from build123d import *

# Parameters (mm, degrees)
SKETCH_1_W      = 80
SKETCH_1_H      = 80
SKETCH_1_R      = 22.5
EXTRUDE_1_DEPTH = 15
FILLET_1_R      = 5
SKETCH_2_R      = 7.5
EXTRUDE_2_DEPTH = 70
FILLET_2_R      = 3


with BuildPart() as part:
    # 草圖1 → 填料-伸長1 (new body)
    with BuildSketch(Plane(origin=(0, 0, 0), x_dir=(1, 0, 0), z_dir=(0, 1, 0))):
        with Locations((11.024390244, -21.451219512)):
            Rectangle(SKETCH_1_W, SKETCH_1_H)
        with Locations(Location((11.024390244, -21.451219512, 0), (0, 0, 270))):
            Circle(SKETCH_1_R, mode=Mode.SUBTRACT)
    extrude(amount=EXTRUDE_1_DEPTH)

    # 圓角1
    fillet_1_edges = [part.edges().sort_by_distance(p)[0] for p in [
        (-28.975609756, 7.5, -18.548780488),
        (51.024390244, 7.5, -18.548780488),
        (51.024390244, 7.5, 61.451219512),
        (-28.975609756, 7.5, 61.451219512),
    ]]
    fillet(fillet_1_edges, radius=FILLET_1_R)

    # 草圖2 → 填料-伸長2 (add)
    with BuildSketch(Plane(origin=(0, 15, 0), x_dir=(1, 0, 0), z_dir=(0, 1, 0))):
        with Locations(Location((-16.475609756, 6.048780488, 0), (0, 0, 270))):
            Circle(SKETCH_2_R)
        with Locations(Location((38.524390244, 6.048780488, 0), (0, 0, 270))):
            Circle(SKETCH_2_R)
        with Locations(Location((38.524390244, -48.951219512, 0), (0, 0, 270))):
            Circle(SKETCH_2_R)
        with Locations(Location((-16.475609756, -48.951219512, 0), (0, 0, 270))):
            Circle(SKETCH_2_R)
    extrude(amount=EXTRUDE_2_DEPTH)

    # 圓角2
    fillet_2_edges = [part.edges().sort_by_distance(p)[0] for p in [
        (-16.475609756, 15, -13.548780488),
        (38.524390244, 15, -13.548780488),
        (38.524390244, 15, 41.451219512),
        (-16.475609756, 15, 41.451219512),
    ]]
    fillet(fillet_2_edges, radius=FILLET_2_R)


solid = part.part
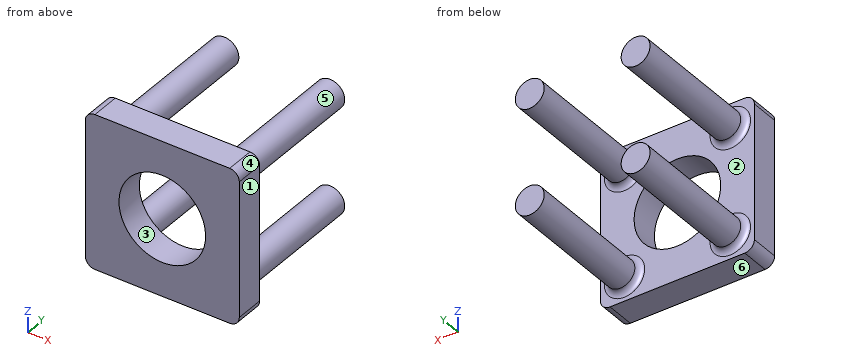
The listing builds one solid part. Answer for the finished solid, in the listing's coordinates (mm). Face numbers are marked on the shaded views. A direction names the side the tool comes from. Coordinates: 2 decimals unless noted, no trailing zeros. Write each loop counter-clockwise with the first axis right and the second up, starting at its lowest first coordinate (ties: lowest second). Pieces come first, ordered by that corner, then holes. Notation, with made-up numbers: (67.25, 31) -> (85.25, 31) arc R27 ccw to (85.25, 55) -> close; hole circle Ø1 at (59.5, -30). An arc over 180 degrees is marked (long way). One line per question, with ' | ' between items.
1. Section C-C (y = 80) is taken. Determine the outline of the cut face in (x, z).
Verdict:
outline: circle Ø15 at (-16.48, -6.05); circle Ø15 at (-16.48, 48.95); circle Ø15 at (38.52, -6.05); circle Ø15 at (38.52, 48.95)
2. Which of the six approach directions +Z, -Z, +X, -X, +Y, -Y give full straight-line access (tool end or side, diameter ignored) to the marked faces 1 and 2?
Verdict:
face 1: +Z, -Z, +X, +Y, -Y | face 2: +Y
3. For a pull along X with two mould halves and no side action, classify the marked faces 3, 4, 5 and 6 as released by +X, released by -X, zero draft, split by the parting line, or undercut.
Verdict:
face 3: undercut | face 4: released by +X | face 5: undercut | face 6: zero draft
4. Given pin 1 Ø1.5 at (y, z) = (62, -10) entering from -X; pin 2 Ø2 at (x, y) = (-12, 19.5) entering from -Z; pin 3 Ø8 at (x, y) = (-6.5, 30.5) entering from +Z; pin 4 Ø1.5 at (x, z) = (30.5, 27) entering from +Y, each flat-ended and moving along its own axis, determine where each tip first touches the part or whether it passes through.
Verdict:
pin 1: stops at x = -23.26 | pin 2: stops at z = -12.69 | pin 3: stops at z = 53.48 | pin 4: passes through
5. Section A-A (z = 37) is taken. Determine the outline of the cut face in (x, y).
Verdict:
outline: (-28.98, 0) -> (-5.24, 0) -> (-5.24, 15) -> (-28.98, 15) -> close; (27.29, 0) -> (51.02, 0) -> (51.02, 15) -> (27.29, 15) -> close
6. Straight lines are drawn through the part: line 1 (X direction, y = 8, z = 2.5); line 2 (Y direction, x = -6.5, z = 6); line 3 (X direction, y = 39.5, z = -12). For each, find the intervals that lie inside material, in ascending order.
Verdict:
line 1: x = -28.98 to -1.1, 23.15 to 51.02 | line 2: y = 0 to 15 | line 3: x = -21.04 to -11.91, 33.96 to 43.09
7. Section B-B (x = 23.5) is taken. Determine the outline of the cut face in (y, z), and give its area (3 significant figures).
Verdict:
outline: (0, -18.55) -> (15, -18.55) -> (15, 2.73) -> (0, 2.73) -> close; (0, 40.18) -> (15, 40.18) -> (15, 61.45) -> (0, 61.45) -> close | area: 638 mm^2
8. Section D-D (y = 10) is taken. Determine the outline of the cut face in (x, z), and give its area (3 significant figures).
Verdict:
outline: (-28.98, -13.55) arc R5 ccw to (-23.98, -18.55) -> (46.02, -18.55) arc R5 ccw to (51.02, -13.55) -> (51.02, 56.45) arc R5 ccw to (46.02, 61.45) -> (-23.98, 61.45) arc R5 ccw to (-28.98, 56.45) -> close; hole circle Ø45 at (11.02, 21.45) | area: 4,790 mm^2
